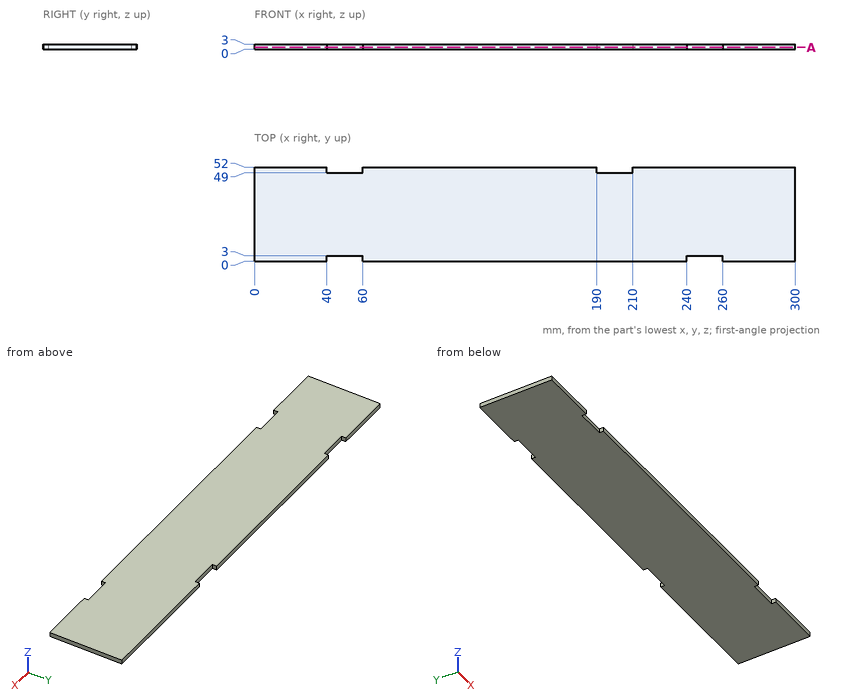
Drawing for the job (mm, zero at the part's lowest x, y, z). Round coordinates to 2 decimals unless told otherwise and drop trailing zeros. Loops run counter-clockwise (first coordinate to the right, second up) from the corner with the lowest first, then second, coordinate; pieces in that order, holes last.
1. Drop a flat-ended pin along its axis: P1, Ø0.9, axis at x = 47.5, z = 1, coming from the -Y side. Give the stop position or say it passes through.
Check values:
P1: stops at y = 3
2. Band-saw the part on A-A, the plane z = 1.15. List the corners of the cut face in (x, y), and give its area (3 significant figures).
Check values:
outline: (0, 0) - (40, 0) - (40, 3) - (60, 3) - (60, 0) - (240, 0) - (240, 3) - (260, 3) - (260, 0) - (300, 0) - (300, 52) - (210, 52) - (210, 49) - (190, 49) - (190, 52) - (60, 52) - (60, 49) - (40, 49) - (40, 52) - (0, 52) - close
area: 15,400 mm2
3. Wall check: probe 1 along Y at (x, z) = (198, 2.35); probe 2 along Y at (x, z) = (42, 2.2). Give the ranges that are in metal, low to high.
Check values:
probe 1: y = 0 to 49
probe 2: y = 3 to 49
